Check sheet for the modelled part. Datum: model origin and axes. Units: mm. A direction names the side the tool comes from. Round coordinates to 2 decimals unless told otherwise and drop trailing zeros. Write each loop counter-clockwise with the first axis right and the second up, starting at its lowest first coordinate (ties: lowest second). Pieces come first, ordered by that corner, then holes.
from build123d import *

# Parameters (mm, degrees)
BOSS_EXTRU_1_DEPTH      = 6
ESQUISSE2_R             = 1.005
ENL_V_MAT_EXTRU_1_DEPTH = 169.277300905
ESQUISSE3_R             = 3
ENL_V_MAT_EXTRU_2_DEPTH = 3
ESQUISSE4_R             = 4
ENL_V_MAT_EXTRU_3_DEPTH = 169.277300905
ESQUISSE5_W             = 27.5
ESQUISSE5_H             = 50
ENL_V_MAT_EXTRU_4_DEPTH = 169.277300905
ESQUISSE6_R             = 3.875
ENL_V_MAT_EXTRU_5_DEPTH = 169.277300905
ESQUISSE7_W             = 10
ESQUISSE7_H             = 50
ENL_V_MAT_EXTRU_6_DEPTH = 169.277300905


with BuildPart() as part:
    # Esquisse1 → Boss.-Extru.1 (new body)
    with BuildSketch(Plane(origin=(0, 0, 0), x_dir=(1, 0, 0), z_dir=(0, 1, 0))):
        Polygon((-159, -32.5), (-159, -10), (-165, -10), (-165, 10), (-159, 10), (-159, 32.5), (159, 32.5), (159, 10), (165, 10), (165, -10), (159, -10), (159, -32.5), align=None)
    extrude(amount=BOSS_EXTRU_1_DEPTH)

    # Esquisse2 → Enlèv. mat.-Extru.1 (cut, through all)
    with BuildSketch(Plane.XZ):
        with Locations(Location((-47.35, 15, 0), (0, 0, 270))):
            Circle(ESQUISSE2_R)
        with Locations(Location((-23.5, 15, 0), (0, 0, 270))):
            Circle(ESQUISSE2_R)
        with Locations(Location((23.5, 15, 0), (0, 0, 90))):
            Circle(ESQUISSE2_R)
        with Locations(Location((47.35, 15, 0), (0, 0, 90))):
            Circle(ESQUISSE2_R)
        with Locations(Location((47.35, -15, 0), (0, 0, 270))):
            Circle(ESQUISSE2_R)
        with Locations(Location((23.5, -15, 0), (0, 0, 270))):
            Circle(ESQUISSE2_R)
        with Locations(Location((-23.5, -15, 0), (0, 0, 90))):
            Circle(ESQUISSE2_R)
        with Locations(Location((-47.35, -15, 0), (0, 0, 90))):
            Circle(ESQUISSE2_R)
        with Locations(Location((0, 15, 0), (0, 0, 270))):
            Circle(ESQUISSE2_R)
        with Locations(Location((0, -15, 0), (0, 0, 90))):
            Circle(ESQUISSE2_R)
    extrude(amount=-ENL_V_MAT_EXTRU_1_DEPTH, mode=Mode.SUBTRACT)

    # Esquisse3 → Enlèv. mat.-Extru.2 (cut)
    with BuildSketch(Plane(origin=(0, 0, 0), x_dir=(-1, 0, 0), z_dir=(0, -1, 0))):
        with Locations(Location((47.35, -15, 0), (0, 0, 90))):
            Circle(ESQUISSE3_R)
        with Locations(Location((23.5, -15, 0), (0, 0, 90))):
            Circle(ESQUISSE3_R)
        with Locations(Location((0, -15, 0), (0, 0, 90))):
            Circle(ESQUISSE3_R)
        with Locations(Location((0, 15, 0), (0, 0, 270))):
            Circle(ESQUISSE3_R)
        with Locations(Location((23.5, 15, 0), (0, 0, 270))):
            Circle(ESQUISSE3_R)
        with Locations(Location((47.35, 15, 0), (0, 0, 270))):
            Circle(ESQUISSE3_R)
        with Locations(Location((-47.35, 15, 0), (0, 0, 90))):
            Circle(ESQUISSE3_R)
        with Locations(Location((-23.5, 15, 0), (0, 0, 90))):
            Circle(ESQUISSE3_R)
        with Locations(Location((-23.5, -15, 0), (0, 0, 270))):
            Circle(ESQUISSE3_R)
        with Locations(Location((-47.35, -15, 0), (0, 0, 270))):
            Circle(ESQUISSE3_R)
    extrude(amount=-ENL_V_MAT_EXTRU_2_DEPTH, mode=Mode.SUBTRACT)

    # Esquisse4 → Enlèv. mat.-Extru.3 (cut, through all)
    with BuildSketch(Plane(origin=(0, 0, 0), x_dir=(-1, 0, 0), z_dir=(0, -1, 0))):
        with Locations(Location((78.5, -21, 0), (0, 0, 90))):
            Circle(ESQUISSE4_R)
        with Locations(Location((-78.5, -21, 0), (0, 0, 270))):
            Circle(ESQUISSE4_R)
        with Locations(Location((78.5, 21, 0), (0, 0, 270))):
            Circle(ESQUISSE4_R)
        with Locations(Location((-78.5, 21, 0), (0, 0, 90))):
            Circle(ESQUISSE4_R)
    extrude(amount=-ENL_V_MAT_EXTRU_3_DEPTH, mode=Mode.SUBTRACT)

    # Esquisse5 → Enlèv. mat.-Extru.4 (cut, through all)
    with BuildSketch(Plane(origin=(0, 0, 0), x_dir=(-1, 0, 0), z_dir=(0, -1, 0))):
        with Locations((102.25, 0)):
            Rectangle(ESQUISSE5_W, ESQUISSE5_H)
        with Locations((-102.25, 0)):
            Rectangle(ESQUISSE5_W, ESQUISSE5_H)
    extrude(amount=-ENL_V_MAT_EXTRU_4_DEPTH, mode=Mode.SUBTRACT)

    # Esquisse6 → Enlèv. mat.-Extru.5 (cut, through all)
    with BuildSketch(Plane(origin=(0, 0, 0), x_dir=(-1, 0, 0), z_dir=(0, -1, 0))):
        with Locations(Location((135, -22, 0), (0, 0, 90))):
            Circle(ESQUISSE6_R)
        with Locations(Location((-135, -22, 0), (0, 0, 270))):
            Circle(ESQUISSE6_R)
        with Locations(Location((-135, 22, 0), (0, 0, 90))):
            Circle(ESQUISSE6_R)
        with Locations(Location((135, 22, 0), (0, 0, 270))):
            Circle(ESQUISSE6_R)
    extrude(amount=-ENL_V_MAT_EXTRU_5_DEPTH, mode=Mode.SUBTRACT)

    # Esquisse7 → Enlèv. mat.-Extru.6 (cut, through all)
    with BuildSketch(Plane(origin=(0, 0, 0), x_dir=(-1, 0, 0), z_dir=(0, -1, 0))):
        with Locations((148, 0)):
            Rectangle(ESQUISSE7_W, ESQUISSE7_H)
        with Locations((-148, 0)):
            Rectangle(ESQUISSE7_W, ESQUISSE7_H)
    extrude(amount=-ENL_V_MAT_EXTRU_6_DEPTH, mode=Mode.SUBTRACT)


solid = part.part
1. Set-up check for faces 1 (the flat face through (-88.5, 3, 0)), 2 (the flat face through (-162, 3, -10)), 3 (the flat face through (47.3, 3, 16.3)): record each of +Z, -Z, +X, -X, +Y, -Y from which the full face is reachable in a straight line by a thin tool's end or side.
2. Go/stop test with flat-tipped pins: pin 1 (3.5 mm diameter, centred on x = 0, z = 15, fed in from -Y); pin 2 (3 mm diameter, centred on y = 2, z = 26, fed in from -X). Record where each tip stops, or that it passes through.
3. Release check for a two-part mould opening along X. For faces 4 (the flat face through (2, 0, 0)), 5 (the cylindrical face through (0, 1, -18)) record: released by +X, released by -X, zero draft, split by the parting line, or undercut.
4. Sectioned sample at D-D, the plane y = 4.7. Give the number of separate pieces and of enclosed holes in the cut face, plus the area to 3 significant figures.
5. Sectioned sample at A-A, the plane x = 135. Enter the section's corners in (y, z) (3 decimals).
6. Scan lines: line 1 along X through (y, z) = (2.4, -5.5); line 2 along Z through (x, y) = (-94.5, 0.95). Record each from-to range of solid material in increasing order.
7. Sectioned sample at C-C, the plane x = 96.5. Enter the section's corners in (y, z), plus the area to 3 significant figures.
8. Sectioned sample at B-B, the plane z = 7. Enter the section's corners in (x, y).
Computed values:
1. face 1: +Y, -Y
1. face 2: -Z, -X, +Y, -Y
1. face 3: -Y
2. pin 1: stops at y = 3
2. pin 2: stops at x = -159
3. face 4: zero draft
3. face 5: undercut
4. separate pieces: 1
4. enclosed holes: 22
4. area: 16,700 mm2
5. outline: (0, -32.5) - (6, -32.5) - (6, -25.875) - (0, -25.875) - close; (0, -18.125) - (6, -18.125) - (6, 18.125) - (0, 18.125) - close; (0, 25.875) - (6, 25.875) - (6, 32.5) - (0, 32.5) - close
6. line 1: x = -165 to -153, -143 to -116, -88.5 to 88.5, 116 to 143, 153 to 165
6. line 2: z = -32.5 to -25, 25 to 32.5
7. outline: (0, -32.5) - (6, -32.5) - (6, -25) - (0, -25) - close; (0, 25) - (6, 25) - (6, 32.5) - (0, 32.5) - close
7. area: 90.0 mm2
8. outline: (-165, 0) - (-153, 0) - (-153, 6) - (-165, 6) - close; (-143, 0) - (-116, 0) - (-116, 6) - (-143, 6) - close; (-88.5, 0) - (88.5, 0) - (88.5, 6) - (-88.5, 6) - close; (116, 0) - (143, 0) - (143, 6) - (116, 6) - close; (153, 0) - (165, 0) - (165, 6) - (153, 6) - close
